```python
from build123d import *
from OCP.BRepFilletAPI import BRepFilletAPI_MakeChamfer

# Parameters (mm, degrees)
SKETCH1_W           = 166.25
SKETCH1_H           = 100
BOSS_EXTRUDE1_DEPTH = 10
SKETCH2_W           = 3.3
SKETCH2_H           = 9.8
BOSS_EXTRUDE2_DEPTH = 166.25
SKETCH3_W           = 3.5
SKETCH3_H           = 109.8
CUT_EXTRUDE1_DEPTH  = 5
CUT_EXTRUDE2_REACH  = 196.122
SKETCH4_R           = 1.9
LPATTERN1_COUNT     = 7
LPATTERN1_PITCH     = 23.75
SKETCH5_W           = 3.5
SKETCH5_H           = 156.25
CUT_EXTRUDE3_DEPTH  = 5
SKETCH6_W           = 146.25
SKETCH6_H           = 85
CUT_EXTRUDE4_DEPTH  = 5
CHAMFER1_SIZE       = 2.5
CHAMFER1_SIZE_2     = 5


with BuildPart() as part:
    # Sketch1 → Boss-Extrude1 (new body)
    with BuildSketch(Plane.YZ):
        with Locations((83.125, 50)):
            Rectangle(SKETCH1_W, SKETCH1_H)
    extrude(amount=-BOSS_EXTRUDE1_DEPTH)

    # Sketch2 → Boss-Extrude2 (add)
    with BuildSketch(Plane(origin=(0, 166.25, 0), x_dir=(-1, 0, 0), z_dir=(0, 1, 0))):
        with Locations((5, -4.9)):
            Rectangle(SKETCH2_W, SKETCH2_H)
    extrude(amount=-BOSS_EXTRUDE2_DEPTH)

    # Sketch3 → Cut-Extrude1 (cut)
    with BuildSketch(Plane(origin=(0, 166.25, 0), x_dir=(-1, 0, 0), z_dir=(0, 1, 0))):
        with Locations((5, 45.1)):
            Rectangle(SKETCH3_W, SKETCH3_H)
    cut_extrude1 = extrude(amount=-CUT_EXTRUDE1_DEPTH, mode=Mode.SUBTRACT)

    # Mirror1: Cut-Extrude1 across plane
    add(cut_extrude1.mirror(Plane.ZX.offset(83.125)), mode=Mode.SUBTRACT)

    # Sketch4 → Cut-Extrude2 (cut, up to next)
    with BuildSketch(Plane.YZ.offset(-3.35), mode=Mode.PRIVATE) as cut_extrude2_sk1:
        with Locations(Location((11.875, -4.9, 0), (0, 0, 270))):
            Circle(SKETCH4_R)
    cut_extrude2_tool1 = extrude(cut_extrude2_sk1.sketch, amount=-CUT_EXTRUDE2_REACH, mode=Mode.PRIVATE) & part.part
    cut_extrude2 = cut_extrude2_tool1.solids().sort_by_distance((-3.35, 11.875, -4.9))[0]
    add(cut_extrude2, mode=Mode.SUBTRACT)

    # LPattern1: Cut-Extrude2 ×7
    with Locations(*[(0, i * LPATTERN1_PITCH, 0) for i in range(1, LPATTERN1_COUNT)]):
        add(cut_extrude2, mode=Mode.SUBTRACT)

    # Sketch5 → Cut-Extrude3 (cut)
    with BuildSketch(Plane.XY.offset(100)):
        with Locations((-5, 83.125)):
            Rectangle(SKETCH5_W, SKETCH5_H)
    extrude(amount=-CUT_EXTRUDE3_DEPTH, mode=Mode.SUBTRACT)

    # Sketch6 → Cut-Extrude4 (cut)
    with BuildSketch(Plane.YZ.offset(-10)):
        with Locations((83.125, 47.5)):
            Rectangle(SKETCH6_W, SKETCH6_H)
    extrude(amount=CUT_EXTRUDE4_DEPTH, mode=Mode.SUBTRACT)

    # Chamfer1
    chamfer1_edges_1 = [part.edges().sort_by_distance(p)[0] for p in [
        (-10, 10, 47.5),
    ]]
    chamfer1_side_1 = [part.faces().sort_by_distance(p)[0] for p in [
        (-10, 9.95, 47.5),
    ]]
    chamfer1_edges_2 = [part.edges().sort_by_distance(p)[0] for p in [
        (-10, 83.125, 5),
    ]]
    chamfer1_side_2 = [part.faces().sort_by_distance(p)[0] for p in [
        (-10, 83.125, 4.95),
    ]]
    chamfer1_edges_3 = [part.edges().sort_by_distance(p)[0] for p in [
        (-10, 156.25, 47.5),
    ]]
    chamfer1_side_3 = [part.faces().sort_by_distance(p)[0] for p in [
        (-10, 156.3, 47.5),
    ]]
    chamfer1_edges_4 = [part.edges().sort_by_distance(p)[0] for p in [
        (-10, 83.125, 90),
    ]]
    chamfer1_side_4 = [part.faces().sort_by_distance(p)[0] for p in [
        (-10, 83.125, 90.05),
    ]]
    chamfer1 = BRepFilletAPI_MakeChamfer(part.part.solid().wrapped)
    for e in chamfer1_edges_1:
        chamfer1.Add(CHAMFER1_SIZE - 0.0001, CHAMFER1_SIZE_2 - 0.0001, e.wrapped, chamfer1_side_1[0].wrapped)
    for e in chamfer1_edges_2:
        chamfer1.Add(CHAMFER1_SIZE - 0.0001, CHAMFER1_SIZE_2 - 0.0001, e.wrapped, chamfer1_side_2[0].wrapped)
    for e in chamfer1_edges_3:
        chamfer1.Add(CHAMFER1_SIZE - 0.0001, CHAMFER1_SIZE_2 - 0.0001, e.wrapped, chamfer1_side_3[0].wrapped)
    for e in chamfer1_edges_4:
        chamfer1.Add(CHAMFER1_SIZE - 0.0001, CHAMFER1_SIZE_2 - 0.0001, e.wrapped, chamfer1_side_4[0].wrapped)
    add(Compound.cast(chamfer1.Shape()), mode=Mode.REPLACE)  # a hair under: the kernel refuses the full size


solid = part.part
```
Geometry check sheet. Reference: the model listing, model coordinates, mm. A direction names the side the tool comes from. Coordinates: 2 decimals unless noted, no trailing zeros. Answer in a Markdown table with one row per item. Add a question column.
1. Section check A-A (z = -4.9). Give the number of separate pieces and of enclosed holes in the cut face, plus the area to 3 significant figures.
2. Draft check along Y on faces 1 (the face through (-2, 166.25, 49)), 2 (the face through (-2, 82, 100)), 3 (the face through (-4.98, 128.77, -4.49)). Enter one of: +Y half, -Y half, draft (parallel to the pull), parting line (faces both ways), or undercut.
3. Access from +Z, -Z, +X, -X, +Y, -Y to the whole of each face (thin tool, end or side, straight path). Record for faces 4 (the face through (-5, 161.25, 43)), 5 (the face through (-2, 82, 0)), 6 (the face through (-5, 82, 48)), 7 (the face through (-8, 82, 100)), 8 (the face through (-6.75, 83, 98)).
4. Gauge pin test, flat ends, axial feed: pin 1 Ø1 at (x, y) = (-9, 74) entering from -Z; pin 2 Ø3 at (y, z) = (59.375, -4.9) entering from -X; pin 3 Ø5 at (y, z) = (35.625, -4.9) entering from -X; pin 4 Ø4.5 at (y, z) = (130.625, -4.9) entering from +X. Record the tip position at first contact, or that the pin passes through.
5. Material ranges on L1, parallel to Z at x = -4.25, y = 46; L2, parallel to X at y = 135.5, z = 56; L3, parallel to Z at x = -6, y = 60, recorded low to high. Write a range as [from, to].
Data:
| question | item | result |
|---|---|---|
| 1 | separate pieces | 8 |
| 1 | enclosed holes | 0 |
| 1 | area | 428 mm² |
| 2 | face 1 | +Y half |
| 2 | face 2 | draft |
| 2 | face 3 | undercut |
| 3 | face 4 | +Z, -Z, +Y |
| 3 | face 5 | -Z, +X, +Y, -Y |
| 3 | face 6 | -X |
| 3 | face 7 | +Z, +X, -X, +Y, -Y |
| 3 | face 8 | +Z |
| 4 | pin 1 | stops at z = 0 |
| 4 | pin 2 | passes through |
| 4 | pin 3 | stops at x = -6.65 |
| 4 | pin 4 | stops at x = -3.35 |
| 5 | L1 | z = [-9.8, 95] |
| 5 | L2 | x = [-5, 0] |
| 5 | L3 | z = [-9.8, -6.69], [-3.11, 4.5], [90.5, 95] |
